Geometry: final body of the model. Coordinates: model frame, mm. A direction names the side the tool comes from. Give positions to 0.01 mm unless a question says otherwise; leave off trailing zeros. Loops run counter-clockwise (first coordinate to the right, second up) from the corner with the lowest first, then second, coordinate; pieces in that order, holes last.
1. Section D-D, the plane z = 8.5. Output: boundary loops of the cut face in (x, y).
2. Material intervals for line 1 along Y through (x, z) = (0, 6.5); line 2 along Y through (x, z) = (-5, 3); line 3 along Y through (x, z) = (0, 2), sorted ascending.
3. Draft query along Y for faces 3 (the face through (0, -52, 5)), 4 (the face through (0.7, -72.15, 6.99)), 5 (the face through (0.7, 72.15, 6.99)), 6 (the face through (47.15, 1.05, 6.99)). Return one class per face: +Y half, -Y half, draft (parallel to the pull), parting line (faces both ways), or undercut.
4. Access query for faces 1 (the face through (-27, 15, 10)), 2 (the face through (32.5, -55, 5)). Directions: +Z, -Z, +X, -X, +Y, -Y. A direction counts if a zero-diameter tool reaches every point of the face in a straight line with its end or side. Return the directions, or none.
5. Section B-B, the plane x = 12. State how many separate pieces and enclosed holes the cut face has, then the cut area to 3 significant figures.
6. First-contact query: P1, Ø6, axis at y = -41.5, z = 6, coming from the +X side; P2, Ø5, axis at y = 4.5, z = 7.5, coming from the +X side; P3, Ø5, axis at x = 12.5, z = 3, coming from the +Y side. Flat tips, straight axial feed; report the tip coordinate or a pass-through.
from build123d import *

# Parameters (mm, degrees)
SKETCH2_W           = 100
SKETCH2_H           = 150
BOSS_EXTRUDE1_DEPTH = 10
FILLET1_R           = 10
SKETCH3_R           = 2.5
CUT_EXTRUDE1_DEPTH  = 10
SKETCH4_W           = 53
SKETCH4_H           = 85
CUT_EXTRUDE2_DEPTH  = 10
SKETCH5_W           = 65
SKETCH5_H           = 6
CUT_EXTRUDE3_DEPTH  = 10


with BuildPart() as part:
    # Sketch2 → Boss-Extrude1 (new body)
    with BuildSketch(Plane.XY):
        Rectangle(SKETCH2_W, SKETCH2_H)
    extrude(amount=BOSS_EXTRUDE1_DEPTH)

    # Fillet1
    fillet1_edges = [part.edges().sort_by_distance(p)[0] for p in [
        (50, 0, 10),
        (0, 75, 10),
        (-50, 0, 10),
        (0, -75, 10),
    ]]
    fillet(fillet1_edges, radius=FILLET1_R - 0.0001)  # a hair under: the kernel refuses the full size

    # Sketch3 → Cut-Extrude1 (cut)
    with BuildSketch(Plane.XY.offset(10)):
        with Locations((0, 50)):
            Circle(SKETCH3_R)
    extrude(amount=-CUT_EXTRUDE1_DEPTH, mode=Mode.SUBTRACT)

    # Sketch4 → Cut-Extrude2 (cut)
    with BuildSketch(Plane.XY.offset(10)):
        Rectangle(SKETCH4_W, SKETCH4_H)
    extrude(amount=-CUT_EXTRUDE2_DEPTH, mode=Mode.SUBTRACT)

    # Sketch5 → Cut-Extrude3 (cut)
    with BuildSketch(Plane.XY.offset(10)):
        with Locations((0, -55)):
            Rectangle(SKETCH5_W, SKETCH5_H)
    extrude(amount=-CUT_EXTRUDE3_DEPTH, mode=Mode.SUBTRACT)


solid = part.part
Answers below:
1. outline: (-45.27, -70.27) - (45.27, -70.27) - (45.27, 70.27) - (-45.27, 70.27) - close; hole (-32.5, -58) - (32.5, -58) - (32.5, -52) - (-32.5, -52) - close; hole (-26.5, -42.5) - (26.5, -42.5) - (26.5, 42.5) - (-26.5, 42.5) - close; hole circle Ø5 at (0, 50)
2. line 1: y = -72.6 to -58, -52 to -42.5, 42.5 to 47.5, 52.5 to 72.6
2. line 2: y = -74.54 to -58, -52 to -42.5, 42.5 to 74.54
2. line 3: y = -74.8 to -58, -52 to -42.5, 42.5 to 47.5, 52.5 to 74.8
3. face 3: undercut
3. face 4: -Y half
3. face 5: +Y half
3. face 6: draft
4. face 1: +Z, +X, -X, +Y, -Y
4. face 2: +Z, -Z
5. separate pieces: 3
5. enclosed holes: 0
5. area: 547 mm2
6. P1: stops at x = 49.54
6. P2: stops at x = 48.66
6. P3: stops at y = 74.99
